Autodesk Inventor part; units mm, degrees
ref_plane "YZ Plane" through (0, 0, 0) normal (1, 0, 0) x (0, 1, 0)
ref_plane "XZ Plane" through (0, 0, 0) normal (0, 1, 0) x (-1, 0, 0)
ref_plane "XY Plane" through (0, 0, 0) normal (0, 0, 1) x (1, 0, 0)
sketch "Sketch1" plane through (0, 0, 0) normal (0, 0, 1) x (1, 0, 0)
  line L0 (-3, -12.5) -> (3, -12.5)
  line L1 (3, -12.5) -> (3, 12.5)
  line L2 (3, 12.5) -> (-3, 12.5)
  line L3 (-3, 12.5) -> (-3, -12.5)
  line L4 (-3, -12.5) -> (3, 12.5) construction
  line L5 (3, -12.5) -> (-3, 12.5) construction
  line L6 (-2, -12.5) -> (2, -12.5)
  line L7 (2, -12.5) -> (2, -15.5)
  line L8 (2, -15.5) -> (-2, -15.5)
  line L9 (-2, -15.5) -> (-2, -12.5)
  line L10 (-2, 7.5) -> (2, 7.5)
  line L11 (2, 7.5) -> (2, 10.5)
  line L12 (2, 10.5) -> (-2, 10.5)
  line L13 (-2, 10.5) -> (-2, 7.5)
  line L14 (-2, 7.5) -> (2, 10.5) construction
  line L15 (2, 7.5) -> (-2, 10.5) construction
  point P0 (0, 0)
  point P1 (0, -15.5)
  point P2 (0, -12.5)
  point P3 (0, 9)
  point P4 (0, 10.5)
  point P5 (0, 12.5)
  dimension "d0" = 25
  dimension "d1" = 6
  dimension "d2" = 3
  dimension "d3" = 4
  dimension "d6" = 4
  dimension "d7" = 3
  dimension "d8" = 2
extrude "Extrusion1" add sketch "Sketch1" along normal blind 3
properties material "MDF Medium Density Fiberboard"
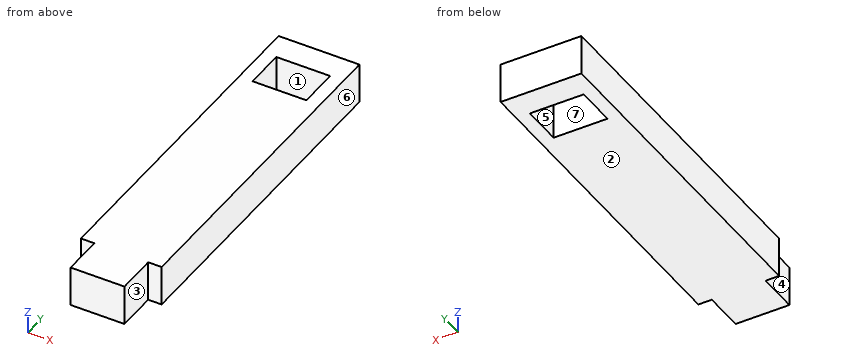
Can you work these out from the model? Positions are in its coordinate system, mm. Face numbers are marked on the shaded views. A direction names the side the tool comes from. Round coordinates to 2 decimals unless told otherwise and drop trailing zeros. Loops run counter-clockwise (first coordinate to the right, second up) from the corner with the lowest first, then second, coordinate; pieces in that order, holes last.
Item 1: Suppose I cut it at D-D, the plane x = 2.55. Write out the boundary of the cut face in (y, z), then the cut area to 3 significant figures.
Item 2: Which directions (+Z, -Z, +X, -X, +Y, -Y) give clear straight access to the entire face, cutting with the end or side of a thin tool? Please do the marked faces 1, 2 and 3.
Item 3: Please list where these lines run through material, in increasing order: L1, parallel to Y at x = 0.85, z = 1.5; L2, parallel to X at y = 8, z = 2.45; L3, parallel to Y at x = 2.25, z = 0.5.
Item 4: Suppose I cut it at C-C, the plane y = 10. Write out the boundary of the cut face in (x, z), then the cut area to 3 significant figures.
Item 5: Will these pins go through, and if not, where does the flat tip stop? pin 1 Ø0.5 at (x, z) = (2.5, 2) entering from -Y; pin 2 Ø1.5 at (y, z) = (-14.5, 1.5) entering from +X.
Item 6: If we mould it in two halves opening along X, with no side actions, what happens to the marked faces 4, 5, 6 and 7? For each: +X half, -X half, draft (parallel to the pull), parting line (faces both ways), or undercut.
Item 7: Suppose I cut it at B-B, the plane z = 1.95. Write out the boundary of the cut face in (x, y), then the cut area to 3 significant figures.
Item 8: Suppose I cut it at A-A, the plane x = 0.6. Write out the boundary of the cut face in (y, z).
Reported:
1. outline: (-12.5, 0) - (12.5, 0) - (12.5, 3) - (-12.5, 3) - close
1. area: 75.0 mm2
2. face 1: +Z, -Z
2. face 2: -Z, +X, -X, +Y, -Y
2. face 3: +Z, -Z, +X, -Y
3. L1: y = -15.5 to 7.5, 10.5 to 12.5
3. L2: x = -3 to -2, 2 to 3
3. L3: y = -12.5 to 12.5
4. outline: (-3, 0) - (-2, 0) - (-2, 3) - (-3, 3) - close; (2, 0) - (3, 0) - (3, 3) - (2, 3) - close
4. area: 6.00 mm2
5. pin 1: stops at y = -12.5
5. pin 2: stops at x = 2
6. face 4: -X half
6. face 5: undercut
6. face 6: +X half
6. face 7: undercut
7. outline: (-3, -12.5) - (-2, -12.5) - (-2, -15.5) - (2, -15.5) - (2, -12.5) - (3, -12.5) - (3, 12.5) - (-3, 12.5) - close; hole (-2, 7.5) - (2, 7.5) - (2, 10.5) - (-2, 10.5) - close
7. area: 150 mm2
8. outline: (-15.5, 0) - (7.5, 0) - (7.5, 3) - (-15.5, 3) - close; (10.5, 0) - (12.5, 0) - (12.5, 3) - (10.5, 3) - close
